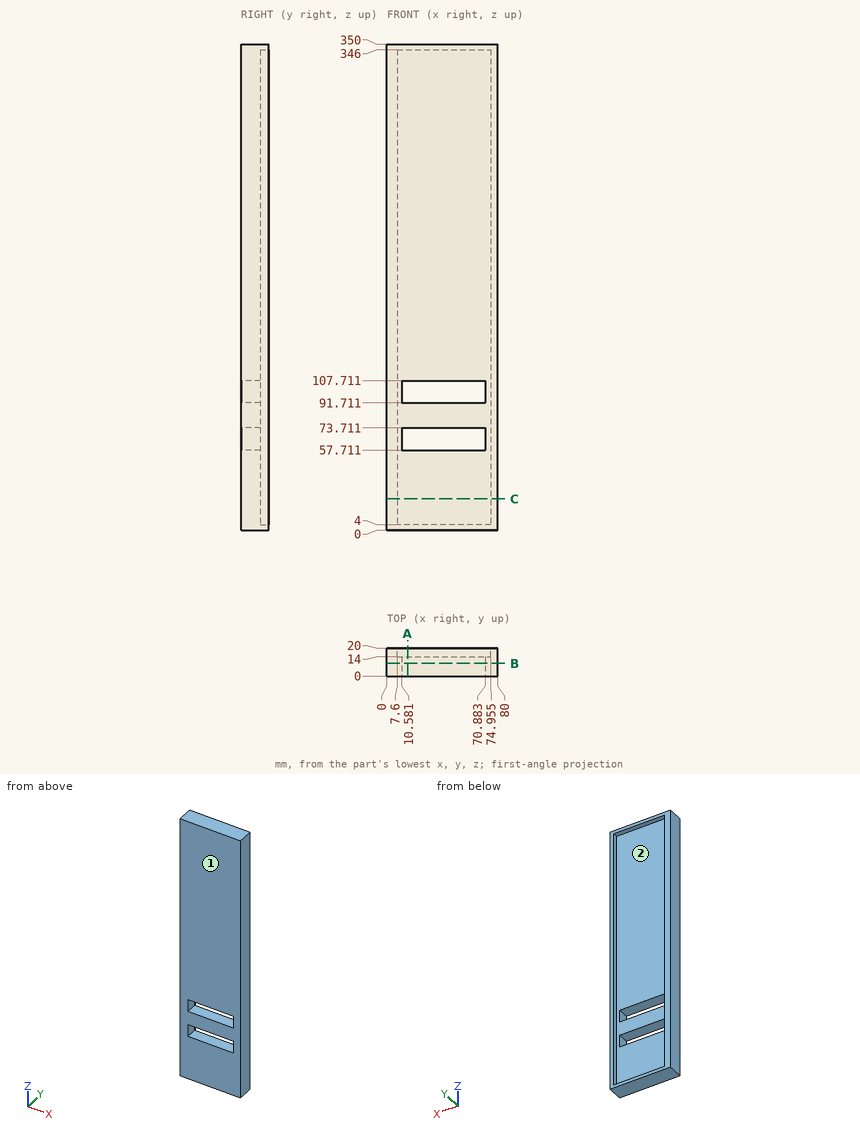
The drawing under review shows one solid part. Ordinate dimensions are in mm from its lowest x, y, z. Give positions to 0.01 mm unless a question says otherwise; leave off trailing zeros. Write each loop counter-clockwise with the first axis right and the second up, starting at its lowest first coordinate (ties: lowest second). Pieces come first, ordered by that corner, then holes. Notation, with made-up numbers: (36.25, 32) -> (93.25, 32) arc R10 ccw to (93.25, 50) -> close; hole circle Ø9 at (80.5, -28.5). An arc over 180 degrees is marked (long way). Answer in a Markdown table with one row per item.
(1) Consider section C-C (z = 22.5). State the section outline as (x, y) points (1 decimal).
Results:
| item | result |
|---|---|
| outline | (0, 0) -> (80, 0) -> (80, 20) -> (75, 20) -> (75, 14) -> (7.6, 14) -> (7.6, 20) -> (0, 20) -> close |
(2) To check wall thickness, follow probe 1 along Z at (x, y) = (54, 2.25); probe 2 along X at (y, z) = (16, 294) (1 decimal); probe 3 along Z at (x, y) = (10, 18.5). State the ranges of each line that lie inside material, in increasing order.
Results:
| item | result |
|---|---|
| probe 1 | 0 to 57.71, 73.71 to 91.71, 107.71 to 350 |
| probe 2 | 0 to 7.6, 75 to 80 |
| probe 3 | 0 to 4, 346 to 350 |
(3) Mouldability with a two-part tool opening along Z and no side actions: class the marked faces 1 and 2 as +Z half, -Z half, draft (parallel to the pull), parting line (faces both ways), or undercut.
Results:
| item | result |
|---|---|
| face 1 | draft |
| face 2 | undercut |
(4) Consider section B-B (y = 9). State the section outline as (x, z) points, then the cut area to 3 significant figures.
Results:
| item | result |
|---|---|
| outline | (0, 0) -> (80, 0) -> (80, 350) -> (0, 350) -> close; hole (10.58, 57.71) -> (70.88, 57.71) -> (70.88, 73.71) -> (10.58, 73.71) -> close; hole (10.58, 91.71) -> (70.88, 91.71) -> (70.88, 107.71) -> (10.58, 107.71) -> close |
| area | 26,100 mm2 |
(5) Consider section A-A (x = 15). State the section outline as (y, z) points.
Results:
| item | result |
|---|---|
| outline | (0, 0) -> (20, 0) -> (20, 4) -> (14, 4) -> (14, 57.71) -> (0, 57.71) -> close; (0, 73.71) -> (14, 73.71) -> (14, 91.71) -> (0, 91.71) -> close; (0, 107.71) -> (14, 107.71) -> (14, 346) -> (20, 346) -> (20, 350) -> (0, 350) -> close |
(6) Clearance check with a flat-ended pin moving along its axis: pin 1 (20 mm diameter, centred on x = 56, z = 158, fed in from +Y). State where the tip first meets the part, or that it passes through.
Results:
| item | result |
|---|---|
| pin 1 | y = 14 |
